Answer from the drawing. Dimensions are ordinates in mm from the lowest x, y and z of the part. Coordinates: 2 decimals unless noted, no trailing zeros. Write each loop counter-clockwise with the first axis right and the second up, starting at its lowest first coordinate (ties: lowest second). Pieces come first, ordered by that corner, then holes. Notation, with made-up numbers: (71, 54.25) - (125, 54.25) arc R17 cw to (125, 68.25) - close; hole circle Ø2 at (19.5, 27). An arc over 180 degrees is marked (long way). Use one line per item in the form item = value. Start each with the question number.
Item 1: A cutting plane is placed at A-A (y = 244.5). Write down the section's boundary in (x, z).
Item 2: A cutting plane is placed at C-C (x = 972). Write down the section's boundary in (y, z).
Item 3: A cutting plane is placed at B-B (z = 869.5). Write down the section's boundary in (x, y), then the cut area to 4 significant figures.
Item 4: Given pin 1 (5 mm diameter, centred on x = 851.5, z = 689, fed in from -Y), flat-ended and moving along its own axis, determine where the tip first touches the part or whether it passes through.
Item 5: Consider probe 1 along Z at (x, y) = (1198.5, 92.5); probe 2 along X at (y, z) = (54, 931); probe 3 along Y at (x, z) = (886.5, 66.5). Determine where each line is inside the solid, lowest interval first.
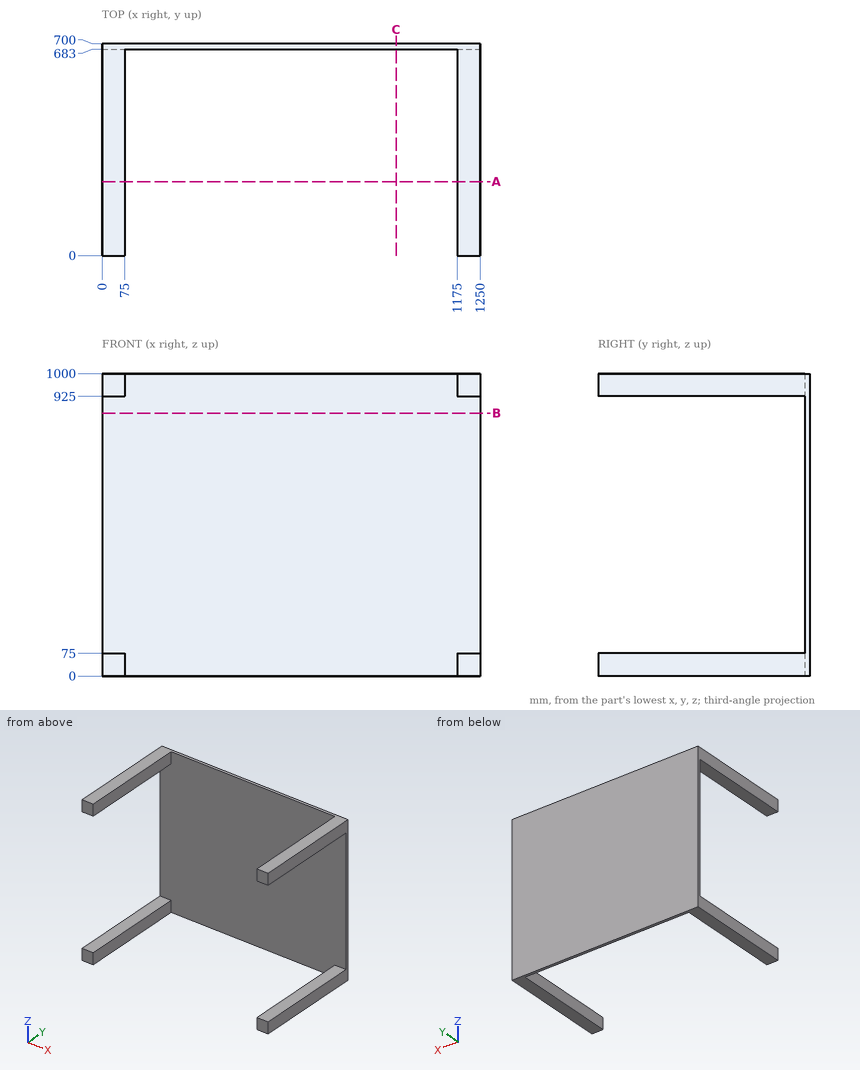
Answer:
q1.outline = (0, 0) - (75, 0) - (75, 75) - (0, 75) - close; (0, 925) - (75, 925) - (75, 1000) - (0, 1000) - close; (1175, 0) - (1250, 0) - (1250, 75) - (1175, 75) - close; (1175, 925) - (1250, 925) - (1250, 1000) - (1175, 1000) - close
q2.outline = (683, 0) - (700, 0) - (700, 1000) - (683, 1000) - close
q3.outline = (0, 683) - (1250, 683) - (1250, 700) - (0, 700) - close
q3.area = 21,250 mm²
q4.pin_1 = 683
q5.probe_1 = 0 to 75, 925 to 1000
q5.probe_2 = 0 to 75, 1175 to 1250
q5.probe_3 = 683 to 700
